Model file for the job. Use its own axes, mm. A direction names the side the tool comes from. Give positions to 0.01 mm unless a question says otherwise; leave off trailing zeros. Loops run counter-clockwise (first coordinate to the right, second up) from the corner with the lowest first, then second, coordinate; pieces in that order, holes last. Notation, with made-up numbers: (-23.75, -38.5) - (10.25, -38.5) arc R27 cw to (10.25, -16.5) - close; hole circle Ø3 at (16.5, 40.5). An arc over 180 degrees is marked (long way). Use a Markdown table: item, result.
from build123d import *

# Parameters (mm, degrees)
SKETCH2_R               = 1.5875
BOSS_EXTRUDE1_DEPTH     = 12.7
CUT_EXTRUDE3_DEPTH      = 12.7
CUT_EXTRUDE3_DEPTH_BACK = 12.7
SKETCH4_W               = 3.175
SKETCH4_H               = 5.378529074
SKETCH4_W_2             = 3.429175225
FILLET4_R               = 0.635
SCALE1_SCALE            = 3


with BuildPart() as part:
    # Sketch2 → Boss-Extrude1 (new body)
    with BuildSketch(Plane(origin=(0, 0, 0), x_dir=(0, 0, -1), z_dir=(1, 0, 0))):
        with BuildLine():
            Line((0.7234417, 2.689264537), (0.7234417, 38.281333312))
            Line((0.7234417, 38.281333312), (2.2225, 38.281333312))
            Line((2.2225, 38.281333312), (2.2225, 0))
            ThreePointArc((2.2225, 0), (-1.641425032, -1.498409194), (0.202045455, 2.213297062))
            ThreePointArc((0.202045455, 2.213297062), (0.567726646, 2.33627761), (0.7234417, 2.689264537))
        make_face()
        Circle(SKETCH2_R, mode=Mode.SUBTRACT)
    extrude(amount=BOSS_EXTRUDE1_DEPTH)

    # Sketch4 → Cut-Extrude3 (cut, two sides: drawn at the far end of the back side and taken through both)
    with BuildSketch(Plane.XY.offset(-0.7234417).offset(-CUT_EXTRUDE3_DEPTH_BACK)):
        with Locations((1.5875, 0)):
            Rectangle(SKETCH4_W, SKETCH4_H)
        with Locations((11.239587612, 0)):
            Rectangle(SKETCH4_W_2, SKETCH4_H)
    extrude(amount=CUT_EXTRUDE3_DEPTH + CUT_EXTRUDE3_DEPTH_BACK, mode=Mode.SUBTRACT)

    # Fillet4
    fillet4_edges = [part.edges().sort_by_distance(p)[0] for p in [
        (12.7, 20.485298925, -0.7234417),
        (0, 20.485298925, -0.7234417),
    ]]
    fillet(fillet4_edges, radius=FILLET4_R)


with BuildPart() as part_1:
    # Scale1: scaled about (6.35, 18.844068161, -1.382882034)
    add(part.part.scale(SCALE1_SCALE).moved(Location((-12.7, -37.688136322, 2.765764068))))


solid = part_1.part
(1) Pin check, flat tips, straight feed: P1, Ø6, axis at x = -8.5, y = -29.5, coming from the +Z side; P2, Ø5, axis at x = 22, z = -1, coming from the -Y side; P3, Ø2, axis at y = 24.5, z = 2, coming from the +X side; P4, Ø1.5, axis at x = 5, z = 5.5, coming from the +Y side. Stop position of each tip, or through.
Computed:
| item | result |
|---|---|
| P1 | z = 0.6 |
| P2 | y = -29.62 |
| P3 | through |
| P4 | y = -31.32 |
(2) 3-axis set-ups, long thin cutter, end or side, ignore diameter. For faces 1 (the flat face through (15.875, -33.8, -0.3)), 2 (the flat face through (-3.175, -33.8, -0.3)), 3 (the flat face through (6, 23, 0.595)), 4 (the cylindrical face through (6.217, -42.346, 7.536)): which of +Z, -Z, +X, -X, +Y, -Y reach the whole face in a straight line?
Computed:
| item | result |
|---|---|
| face 1 | +Z, -Z, +X, -Y |
| face 2 | +Z, -Z, -X, -Y |
| face 3 | +Z, +X, -X, +Y |
| face 4 | +X, -X |
(3) Slice it at B-B, the plane y = 68. Write the cut outline in (x, z) (3 decimals).
Computed:
| item | result |
|---|---|
| outline | (-12.7, -3.902) - (25.4, -3.902) - (25.4, -1.31) arc R1.905 ccw to (23.495, 0.595) - (-10.795, 0.595) arc R1.905 ccw to (-12.7, -1.31) - close |
(4) Slice it at D-D, the plane x = 2. Write the cut outline in (y, z) (1 decimal), plus the area to 3 significant figures.
Computed:
| item | result |
|---|---|
| outline | (-37.7, -3.9) - (77.2, -3.9) - (77.2, 0.6) - (-29.6, 0.6) arc R1.4 cw to (-31, 2.2) arc R6.7 ccw (long way) to start; hole circle Ø9.5 at (-37.7, 2.8) |
| area | 565 mm² |
(5) Mould opens along Y. For faces 5 (the cylindrical face through (6.22, -33.67, 0.21)), 6 (the flat face through (-12.7, 25, -3)), 7 (the flat face through (-8, -29.62, -2)) say: pulls with the +Y half, pulls with the -Y half, needs draft (parallel to the pull), parting line crosses it, or undercut.
Computed:
| item | result |
|---|---|
| face 5 | undercut |
| face 6 | needs draft |
| face 7 | pulls with the -Y half |
(6) Slice it at C-C, the plane x = 18. Write the cut outline in (y, z), plus the area to 3 significant figures.
Computed:
| item | result |
|---|---|
| outline | (-29.62, -3.9) - (77.16, -3.9) - (77.16, 0.6) - (-29.62, 0.6) - close |
| area | 480 mm² |
(7) Slice it at A-A, the plane z = 5.5. Write the cut outline in (x, y) (3 decimals), plus the area to 3 significant figures.
Computed:
| item | result |
|---|---|
| outline | (-3.175, -43.769) - (15.875, -43.769) - (15.875, -41.588) - (-3.175, -41.588) - close; (-3.175, -33.789) - (15.875, -33.789) - (15.875, -31.607) - (-3.175, -31.607) - close |
| area | 83.1 mm² |
(8) Drill centre lines: probe 1 along Z at (x, y) = (2, 6.5); probe 2 along Z at (x, y) = (10, -37.5); probe 3 along Y at (x, z) = (10, 2.5). Where is each one in solid material? Low to high. Write a range as [from, to].
Computed:
| item | result |
|---|---|
| probe 1 | [-3.9, 0.6] |
| probe 2 | [-3.9, -1.99], [7.52, 9.43] |
| probe 3 | [-44.35, -42.44], [-32.93, -31.03] |
